For this review, use the dimensioned drawing (mm, ordinates from the lowest corner) and the shaded views. A direction names the side the tool comes from. Coordinates: 2 decimals unless noted, no trailing zeros. Order: outer loops, then holes, each group sorted by start corner. A loop starts at its lowest first (then second) coordinate and runs counter-clockwise, first axis right, second up. Notation, with made-up numbers: M 50.5,84 L 57.5,84 A18 cw 57.5,113 Z; hole C -40,83 d2. An arc over 180 degrees is marked long. One line per item, written item: value.
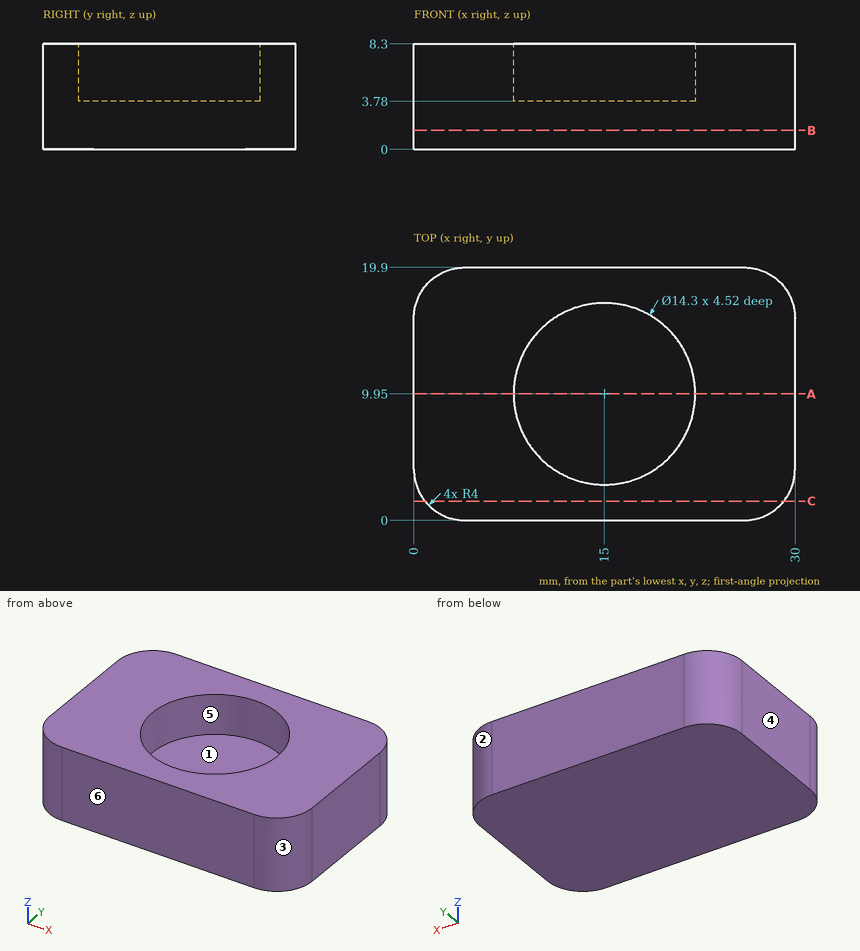
(1) Tool access review of the marked faces 5 and 6: name each direction out of +Z, -Z, +X, -X, +Y, -Y from which nothing blocks a thin tool from reaching the whole face with its end or side.
Geometry results:
face 5: +Z
face 6: +Z, -Z, +X, -X, -Y
(2) We need section B-B, the plane z = 1.5. State the section outline as (x, y) points.
Geometry results:
outline: M 0,4 A4 ccw 4,0 L 26,0 A4 ccw 30,4 L 30,15.9 A4 ccw 26,19.9 L 4,19.9 A4 ccw 0,15.9 Z
(3) Mouldability with a two-part tool opening along Y and no side actions: class the marked faces 1, 2, 3 and 4 as +Y half, -Y half, draft (parallel to the pull), parting line (faces both ways), or undercut.
Geometry results:
face 1: undercut
face 2: +Y half
face 3: -Y half
face 4: draft
(4) We need section C-C, the plane y = 1.5. State the section outline as (x, z) points, plus the area to 3 significant figures.
Geometry results:
outline: M 0.88,0 L 29.12,0 L 29.12,8.3 L 0.88,8.3 Z
area: 234 mm2
(5) We need section A-A, the plane y = 9.95. State the section outline as (x, z) points.
Geometry results:
outline: M 0,0 L 30,0 L 30,8.3 L 22.15,8.3 L 22.15,3.78 L 7.85,3.78 L 7.85,8.3 L 0,8.3 Z
(6) Insertion check: pin 1 Ø4 at (x, y) = (16.5, 14) entering from +Z; pin 2 Ø2 at (x, z) = (15.5, 7.5) entering from -Y. Each pin has a flat end and moves straight along its axis. Give the tip position at first contact, or say it passes through.
Geometry results:
pin 1: stops at z = 3.78
pin 2: stops at y = 0
(7) For L1, parallel to Y at x = 15, z = 6.15; L2, parallel to Z at x = 9, y = 12; L3, parallel to X at y = 6, z = 4, list the stretches that pass through material, from the lowest coordinate up.
Geometry results:
L1: y = 0 to 2.8, 17.1 to 19.9
L2: z = 0 to 3.78
L3: x = 0 to 9.04, 20.96 to 30
